Source: CAD feature listing. Evaluate the final solid. Frame: model axes, mm. A direction names the side the tool comes from. Give positions to 0.01 mm unless a question says otherwise; leave off trailing zeros. Loops run counter-clockwise (first coordinate to the right, second up) from the corner with the lowest first, then second, coordinate; pieces in that order, holes last. Notation, with made-up numbers: M 20.25,-14 L 68.25,-14 A18 cw 68.25,12 Z; hole C 36,70.25 d1. An arc over 180 degrees is marked long. Answer in a Markdown table with one row per item.
```python
from build123d import *

# Parameters (mm, degrees)
SKETCH_1_R      = 1.25
SKETCH_1_R_2    = 11
EXTRUDE_1_DEPTH = 4
SKETCH_2_W      = 28.2
SKETCH_2_H      = 4
SKETCH_2_H_2    = 40
EXTRUDE_2_DEPTH = 4
EXTRUDE_3_DEPTH = 2


with BuildPart() as part:
    # 草图1 → 凸台-拉伸1 (new body)
    with BuildSketch(Plane.XY):
        with BuildLine():
            Line((14.449257035, -14.332751245), (14.449257035, 44.867089431))
            Line((14.449257035, 44.867089431), (-13.750742965, 44.867089431))
            Line((-13.750742965, 44.867089431), (-13.750742965, -14.332751245))
            ThreePointArc((-13.750742965, -14.332751245), (-13.194199184, -15.676366788), (-11.850583641, -16.232910569))
            Line((-11.850583641, -16.232910569), (0.349257035, -16.232910569))
            Line((0.349257035, -16.232910569), (12.549097711, -16.232910569))
            ThreePointArc((12.549097711, -16.232910569), (13.892713254, -15.676366788), (14.449257035, -14.332751245))
        make_face()
        with Locations((-11.150742965, 9.367089431)):
            Circle(SKETCH_1_R, mode=Mode.SUBTRACT)
        with Locations((11.849257035, 9.367089431)):
            Circle(SKETCH_1_R, mode=Mode.SUBTRACT)
        with Locations((-11.150742965, -13.632910569)):
            Circle(SKETCH_1_R, mode=Mode.SUBTRACT)
        with Locations((11.849257035, -13.632910569)):
            Circle(SKETCH_1_R, mode=Mode.SUBTRACT)
        with Locations((0.349257035, -2.132910569)):
            Circle(SKETCH_1_R_2, mode=Mode.SUBTRACT)
    extrude(amount=EXTRUDE_1_DEPTH)

    # 草图2 → 凸台-拉伸2 (add)
    with BuildSketch(Plane(origin=(0, 44.867089431, 0), x_dir=(1, 0, 0), z_dir=(0, 1, 0))):
        with Locations((0.349257035, -2)):
            Rectangle(SKETCH_2_W, SKETCH_2_H)
        with Locations((0.349257035, 20)):
            Rectangle(SKETCH_2_W, SKETCH_2_H_2)
        with BuildLine():
            ThreePointArc((-5.100742965, 6), (-6.700742965, 4.4), (-8.300742965, 6))
            Line((-8.300742965, 6), (-8.300742965, 30))
            ThreePointArc((-8.300742965, 30), (-6.700742965, 31.6), (-5.100742965, 30))
            Line((-5.100742965, 30), (-5.100742965, 6))
        make_face(mode=Mode.SUBTRACT)
        with BuildLine():
            ThreePointArc((8.999257035, 6), (7.399257035, 4.4), (5.799257035, 6))
            Line((5.799257035, 6), (5.799257035, 30))
            ThreePointArc((5.799257035, 30), (7.399257035, 31.6), (8.999257035, 30))
            Line((8.999257035, 30), (8.999257035, 6))
        make_face(mode=Mode.SUBTRACT)
    extrude(amount=EXTRUDE_2_DEPTH)

    # 草图3 → 凸台-拉伸3 (add)
    with BuildSketch(Plane(origin=(14.449257035, 0, 0), x_dir=(0, 0, -1), z_dir=(1, 0, 0))):
        Polygon((20, 44.867089431), (0, 44.867089431), (0, 24.867089431), align=None)
    extrude_3 = extrude(amount=-EXTRUDE_3_DEPTH)

    # 镜向2: 凸台-拉伸3 across plane
    add(extrude_3.mirror(Plane(origin=(0.349257035, 0, 0), x_dir=(0, 0, 1), z_dir=(1, 0, 0))))


solid = part.part
```
Q1. Mould query, pull axis X, two halves, no side actions, for faces 1 (the flat face through (0, 48.867, -18)), 2 (the cylindrical face through (-13.21, -15.66, 1.97)), 3 (the cylindrical face through (-6.7, 46.8, -31.6)). Classes: +X half, -X half, draft (parallel to the pull), parting line (faces both ways), or undercut.
Values follow:
| item | result |
|---|---|
| face 1 | draft |
| face 2 | -X half |
| face 3 | undercut |
Q2. Section query D-D (z = 1). Output: boundary loops of the cut face in (x, y), plus the area to 3 significant figures.
Values follow:
| item | result |
|---|---|
| outline | M -13.75,-14.33 A1.9 ccw -11.85,-16.23 L 12.55,-16.23 A1.9 ccw 14.45,-14.33 L 14.45,48.87 L -13.75,48.87 Z; hole C -11.15,-13.63 d2.5; hole C -11.15,9.37 d2.5; hole C 0.35,-2.13 d22; hole C 11.85,-13.63 d2.5; hole C 11.85,9.37 d2.5 |
| area | 1,430 mm^2 |
Q3. Reachability of faces 4 (the flat face through (5.799, 47, -18)), 5 (the cylindrical face through (13.004, 8.888, 1.972)), 6 (the flat face through (0, 44.867, -20)) from +Z, -Z, +X, -X, +Y, -Y: full face, straight path, thin tool, end or side. Return the list, or none.
Values follow:
| item | result |
|---|---|
| face 4 | +Y, -Y |
| face 5 | +Z, -Z |
| face 6 | -Z, -Y |
Q4. Section query B-B (z = -16). Output: boundary loops of the cut face in (x, y), plus the area to 3 significant figures.
Values follow:
| item | result |
|---|---|
| outline | M -13.75,40.87 L -11.75,40.87 L -11.75,44.87 L -8.3,44.87 L -8.3,48.87 L -13.75,48.87 Z; M -5.1,44.87 L 5.8,44.87 L 5.8,48.87 L -5.1,48.87 Z; M 9,44.87 L 12.45,44.87 L 12.45,40.87 L 14.45,40.87 L 14.45,48.87 L 9,48.87 Z |
| area | 103 mm^2 |
Q5. Contact query for flat-ended pins moving along their axis: pin 1 Ø2 at (x, y) = (11.85, 9.37) entering from +Z; pin 2 Ø14 at (x, z) = (7.5, -17.5) entering from -Y; pin 3 Ø12 at (x, y) = (-9, -5.5) entering from -Z; pin 4 Ø4 at (x, z) = (5.5, -18.5) entering from -Y. Output: stop coordinate, or through.
Values follow:
| item | result |
|---|---|
| pin 1 | through |
| pin 2 | y = 37.42 |
| pin 3 | z = 0 |
| pin 4 | y = 44.87 |
Q6. Section query C-C (x = -9). Output: boundary loops of the cut face in (y, z), plus the area to 3 significant figures.
Values follow:
| item | result |
|---|---|
| outline | M -16.23,0 L -7.93,0 L -7.93,4 L -16.23,4 Z; M 3.66,0 L 44.87,0 L 44.87,-40 L 48.87,-40 L 48.87,4 L 3.66,4 Z |
| area | 374 mm^2 |
Q7. Section query A-A (y = -8.5). Output: boundary loops of the cut face in (x, z), plus the area to 3 significant figures.
Values follow:
| item | result |
|---|---|
| outline | M -13.75,0 L -8.62,0 L -8.62,4 L -13.75,4 Z; M 9.32,0 L 14.45,0 L 14.45,4 L 9.32,4 Z |
| area | 41.0 mm^2 |
Q8. Ray query, probe 1 along X at (y, z) = (36, -2); probe 2 along Z at (x, y) = (-11, 3); probe 3 along Y at (x, z) = (10.5, -4). Return the intervals inside material, ascending. Write a range as from..to.
Values follow:
| item | result |
|---|---|
| probe 1 | -13.75..-11.75, 12.45..14.45 |
| probe 2 | 0..4 |
| probe 3 | 44.87..48.87 |
